```python
from build123d import *

# Parameters (mm, degrees)
CROQUIS1_W              = 32.64
CROQUIS1_H              = 72
CROQUIS1_R              = 1.435
SALIENTE_EXTRUIR4_DEPTH = 4
CROQUIS3_W              = 9
CROQUIS3_H              = 8
CROQUIS3_R              = 1.5
SALIENTE_EXTRUIR5_DEPTH = 4
CROQUIS6_W              = 5.968272271
CROQUIS6_H              = 30
SALIENTE_EXTRUIR6_DEPTH = 4
CROQUIS5_W              = 2.2
CROQUIS5_H              = 50.2
CROQUIS5_H_2            = 30
CORTAR_EXTRUIR1_DEPTH   = 4


with BuildPart() as part:
    # Croquis1 → Saliente-Extruir4 (new body)
    with BuildSketch(Plane.XY):
        with Locations((16.32, 36)):
            Rectangle(CROQUIS1_W, CROQUIS1_H)
        with Locations((2.005, 69.99)):
            Circle(CROQUIS1_R, mode=Mode.SUBTRACT)
        with Locations((2.005, 2.01)):
            Circle(CROQUIS1_R, mode=Mode.SUBTRACT)
        with Locations(Location((30.635, 2.01, 0), (0, 0, 180))):
            Circle(CROQUIS1_R, mode=Mode.SUBTRACT)
        with Locations(Location((30.635, 69.99, 0), (0, 0, 180))):
            Circle(CROQUIS1_R, mode=Mode.SUBTRACT)
        with BuildLine():
            Line((15.32, 3.01), (15.32, 35))
            Line((15.32, 35), (13.49, 35))
            Line((13.49, 35), (13.49, 34))
            Line((13.49, 34), (13.49, 7.851322515))
            ThreePointArc((13.49, 7.851322515), (12.49, 6.851322515), (11.49, 7.851322515))
            Line((11.49, 7.851322515), (11.49, 34))
            Line((11.49, 34), (11.49, 35))
            Line((11.49, 35), (9.66, 35))
            Line((9.66, 35), (9.66, 34))
            Line((9.66, 34), (9.66, 13.772536222))
            ThreePointArc((9.66, 13.772536222), (8.66, 12.772536222), (7.66, 13.772536222))
            Line((7.66, 13.772536222), (7.66, 34))
            Line((7.66, 34), (7.66, 35))
            Line((7.66, 35), (5.83, 35))
            Line((5.83, 35), (5.83, 34))
            Line((5.83, 34), (5.83, 23.099052443))
            ThreePointArc((5.83, 23.099052443), (4.83, 22.099052443), (3.83, 23.099052443))
            Line((3.83, 23.099052443), (3.83, 34))
            Line((3.83, 34), (3.83, 35))
            Line((3.83, 35), (3.005, 35))
            ThreePointArc((3.005, 35), (2.005, 36), (3.005, 37))
            Line((3.005, 37), (3.83, 37))
            Line((3.83, 37), (3.83, 38))
            Line((3.83, 38), (3.83, 48.900947557))
            ThreePointArc((3.83, 48.900947557), (4.83, 49.900947557), (5.83, 48.900947557))
            Line((5.83, 48.900947557), (5.83, 38))
            Line((5.83, 38), (5.83, 37))
            Line((5.83, 37), (7.66, 37))
            Line((7.66, 37), (7.66, 38))
            Line((7.66, 38), (7.66, 58.227463778))
            ThreePointArc((7.66, 58.227463778), (8.66, 59.227463778), (9.66, 58.227463778))
            Line((9.66, 58.227463778), (9.66, 38))
            Line((9.66, 38), (9.66, 37))
            Line((9.66, 37), (11.49, 37))
            Line((11.49, 37), (11.49, 38))
            Line((11.49, 38), (11.49, 64.148677485))
            ThreePointArc((11.49, 64.148677485), (12.49, 65.148677485), (13.49, 64.148677485))
            Line((13.49, 64.148677485), (13.49, 38))
            Line((13.49, 38), (13.49, 37))
            Line((13.49, 37), (15.32, 37))
            Line((15.32, 37), (15.32, 68.99))
            ThreePointArc((15.32, 68.99), (16.32, 69.99), (17.32, 68.99))
            Line((17.32, 68.99), (17.32, 37))
            Line((17.32, 37), (19.15, 37))
            Line((19.15, 37), (19.15, 38))
            Line((19.15, 38), (19.15, 64.148677485))
            ThreePointArc((19.15, 64.148677485), (20.15, 65.148677485), (21.15, 64.148677485))
            Line((21.15, 64.148677485), (21.15, 38))
            Line((21.15, 38), (21.15, 37))
            Line((21.15, 37), (22.98, 37))
            Line((22.98, 37), (22.98, 38))
            Line((22.98, 38), (22.98, 58.227463778))
            ThreePointArc((22.98, 58.227463778), (23.98, 59.227463778), (24.98, 58.227463778))
            Line((24.98, 58.227463778), (24.98, 38))
            Line((24.98, 38), (24.98, 37))
            Line((24.98, 37), (26.81, 37))
            Line((26.81, 37), (26.81, 38))
            Line((26.81, 38), (26.81, 48.900947557))
            ThreePointArc((26.81, 48.900947557), (27.81, 49.900947557), (28.81, 48.900947557))
            Line((28.81, 48.900947557), (28.81, 38))
            Line((28.81, 38), (28.81, 37))
            Line((28.81, 37), (29.635, 37))
            ThreePointArc((29.635, 37), (30.635, 36), (29.635, 35))
            Line((29.635, 35), (28.81, 35))
            Line((28.81, 35), (28.81, 34))
            Line((28.81, 34), (28.81, 23.099052443))
            ThreePointArc((28.81, 23.099052443), (27.81, 22.099052443), (26.81, 23.099052443))
            Line((26.81, 23.099052443), (26.81, 34))
            Line((26.81, 34), (26.81, 35))
            Line((26.81, 35), (24.98, 35))
            Line((24.98, 35), (24.98, 34))
            Line((24.98, 34), (24.98, 13.772536222))
            ThreePointArc((24.98, 13.772536222), (23.98, 12.772536222), (22.98, 13.772536222))
            Line((22.98, 13.772536222), (22.98, 34))
            Line((22.98, 34), (22.98, 35))
            Line((22.98, 35), (21.15, 35))
            Line((21.15, 35), (21.15, 34))
            Line((21.15, 34), (21.15, 7.851322515))
            ThreePointArc((21.15, 7.851322515), (20.15, 6.851322515), (19.15, 7.851322515))
            Line((19.15, 7.851322515), (19.15, 34))
            Line((19.15, 34), (19.15, 35))
            Line((19.15, 35), (17.32, 35))
            Line((17.32, 35), (17.32, 3.01))
            ThreePointArc((17.32, 3.01), (16.32, 2.01), (15.32, 3.01))
        make_face(mode=Mode.SUBTRACT)
    extrude(amount=SALIENTE_EXTRUIR4_DEPTH)

    # Croquis3 → Saliente-Extruir5 (add)
    # profile 1 of 2: a face of its own
    with BuildSketch(Plane.XY.offset(4)):
        with Locations((-4.5, 24)):
            Rectangle(CROQUIS3_W, CROQUIS3_H)
        with Locations((-5, 24)):
            Circle(CROQUIS3_R, mode=Mode.SUBTRACT)
    # profile 2 of 2: a face of its own
    with BuildSketch(Plane.XY.offset(4)):
        with Locations((37.14, 24)):
            Rectangle(CROQUIS3_W, CROQUIS3_H)
        with Locations((37.64, 24)):
            Circle(CROQUIS3_R, mode=Mode.SUBTRACT)
    extrude(amount=-SALIENTE_EXTRUIR5_DEPTH)

    # Croquis6 → Saliente-Extruir6 (add)
    with BuildSketch(Plane.XY.offset(4)):
        with Locations((4.675863865, 36)):
            Rectangle(CROQUIS6_W, CROQUIS6_H)
        with Locations((27.964136135, 36)):
            Rectangle(CROQUIS6_W, CROQUIS6_H)
    extrude(amount=-SALIENTE_EXTRUIR6_DEPTH)

    # Croquis5 → Cortar-Extruir1 (cut)
    with BuildSketch(Plane.XY.offset(4)):
        with Locations((2.1, 41.9)):
            Rectangle(CROQUIS5_W, CROQUIS5_H)
        with Locations((30.54, 52)):
            Rectangle(CROQUIS5_W, CROQUIS5_H_2)
    extrude(amount=-CORTAR_EXTRUIR1_DEPTH, mode=Mode.SUBTRACT)


solid = part.part
```
Input: part model. Units: mm. Frame: model coordinates. Round coordinates to 2 decimals unless told otherwise and drop trailing zeros. Loops run counter-clockwise (first coordinate to the right, second up) from the corner with the lowest first, then second, coordinate; pieces in that order, holes last. Notation, with made-up numbers: (-19, -1.5) - (31, -1.5) arc R34 ccw to (31, 34.5) - close; hole circle Ø2 at (-18, 38). An arc over 180 degrees is marked (long way). One line per item, written item: value. Start each with the question number.
(1) Ray query, line 1 (Y direction, x = 11, z = 1.65); line 2 (Y direction, x = 37.64, z = 1.25); line 3 (X direction, y = 36, z = 1.35). Return the intervals inside material, ascending. Write a range as [from, to].
(2) Contact query for flat-ended pins moving along their axis: P1, Ø1, axis at x = 9.5, y = 14, coming from the -Z side; P2, Ø1.2, axis at y = 13.5, z = 1.5, coming from the -X side; P3, Ø1, axis at x = -3, z = 0.5, coming from the +Y side. Output: stop coordinate, or through.
(3) Section D-D, the plane x = 16.32. Return loops of the section in (y, z).
(4) Section B-B, the plane y = 62.5. Return loops of the section in (x, z).
(5) Section A-A, the plane x = 23.98. Return loops of the section in (y, z), plus the area to 3 significant figures.
(6) Section C-C, the plane y = 21. Return loops of the section in (x, z), plus the area to 3 significant figures.
(7) Draft query along Y for faces 1 (the flat face through (37, 28, 2)), 2 (the flat face through (0, 50, 2)), 3 (the flat face through (29.44, 52, 2)). Return one class per face: +Y half, -Y half, draft (parallel to the pull), parting line (faces both ways), or undercut.
Results below:
1. line 1: [0, 35], [37, 72]
1. line 2: [20, 22.5], [25.5, 28]
1. line 3: [0, 1], [3.2, 7.66], [24.98, 32.64]
2. P1: z = 0
2. P2: x = 0
2. P3: y = 28
3. outline: (0, 0) - (2.01, 0) - (2.01, 4) - (0, 4) - close; (69.99, 0) - (72, 0) - (72, 4) - (69.99, 4) - close
4. outline: (0, 0) - (1, 0) - (1, 4) - (0, 4) - close; (3.2, 0) - (11.49, 0) - (11.49, 4) - (3.2, 4) - close; (13.49, 0) - (15.32, 0) - (15.32, 4) - (13.49, 4) - close; (17.32, 0) - (19.15, 0) - (19.15, 4) - (17.32, 4) - close; (21.15, 0) - (29.44, 0) - (29.44, 4) - (21.15, 4) - close; (31.64, 0) - (32.64, 0) - (32.64, 4) - (31.64, 4) - close
5. outline: (0, 0) - (12.77, 0) - (12.77, 4) - (0, 4) - close; (59.23, 0) - (72, 0) - (72, 4) - (59.23, 4) - close
5. area: 102 mm^2
6. outline: (-9, 0) - (1, 0) - (1, 4) - (-9, 4) - close; (3.2, 0) - (7.66, 0) - (7.66, 4) - (3.2, 4) - close; (9.66, 0) - (11.49, 0) - (11.49, 4) - (9.66, 4) - close; (13.49, 0) - (15.32, 0) - (15.32, 4) - (13.49, 4) - close; (17.32, 0) - (19.15, 0) - (19.15, 4) - (17.32, 4) - close; (21.15, 0) - (22.98, 0) - (22.98, 4) - (21.15, 4) - close; (24.98, 0) - (41.64, 0) - (41.64, 4) - (24.98, 4) - close
6. area: 154 mm^2
7. face 1: +Y half
7. face 2: draft
7. face 3: undercut
